```python
from build123d import *

# Parameters (mm, degrees)
BODY_START          = -127.5
SKETCH1_R           = 25
BODY_DEPTH          = 255
END_CAP_IN_START    = -127.5
SKETCH2_R           = 26
END_CAP_IN_DEPTH    = 18
END_CAP_OUT_START   = 109.5
SKETCH3_R           = 26
END_CAP_OUT_DEPTH   = 18
INLET_PORT_START    = -139.5
SKETCH4_R           = 6
INLET_PORT_DEPTH    = 12
INLET_SOCKET_START  = -139.5
SKETCH5_R           = 3.2
INLET_SOCKET_DEPTH  = 10
OUTLET_PORT_START   = 127.5
SKETCH6_R           = 6
OUTLET_PORT_DEPTH   = 12
OUTLET_SOCKET_START = 129.5
SKETCH7_R           = 3.2
OUTLET_SOCKET_DEPTH = 10


with BuildPart() as part:
    # Sketch1 → Body (new body)
    with BuildSketch(Plane(origin=(0, 0, 0), x_dir=(0, 0, -1), z_dir=(1, 0, 0)).offset(BODY_START)):
        Circle(SKETCH1_R)
    extrude(amount=BODY_DEPTH)

    # Sketch2 → End_Cap_In (add)
    with BuildSketch(Plane(origin=(0, 0, 0), x_dir=(0, 0, -1), z_dir=(1, 0, 0)).offset(END_CAP_IN_START)):
        Circle(SKETCH2_R)
    extrude(amount=END_CAP_IN_DEPTH)

    # Sketch3 → End_Cap_Out (add)
    with BuildSketch(Plane(origin=(0, 0, 0), x_dir=(0, 0, -1), z_dir=(1, 0, 0)).offset(END_CAP_OUT_START)):
        Circle(SKETCH3_R)
    extrude(amount=END_CAP_OUT_DEPTH)

    # Sketch4 → Inlet_Port (add)
    with BuildSketch(Plane(origin=(0, 0, 0), x_dir=(0, 0, -1), z_dir=(1, 0, 0)).offset(INLET_PORT_START)):
        Circle(SKETCH4_R)
    extrude(amount=INLET_PORT_DEPTH)

    # Sketch5 → Inlet_Socket (cut)
    with BuildSketch(Plane(origin=(0, 0, 0), x_dir=(0, 0, -1), z_dir=(1, 0, 0)).offset(INLET_SOCKET_START)):
        Circle(SKETCH5_R)
    extrude(amount=INLET_SOCKET_DEPTH, mode=Mode.SUBTRACT)

    # Sketch6 → Outlet_Port (add)
    with BuildSketch(Plane(origin=(0, 0, 0), x_dir=(0, 0, -1), z_dir=(1, 0, 0)).offset(OUTLET_PORT_START)):
        Circle(SKETCH6_R)
    extrude(amount=OUTLET_PORT_DEPTH)

    # Sketch7 → Outlet_Socket (cut)
    with BuildSketch(Plane(origin=(0, 0, 0), x_dir=(0, 0, -1), z_dir=(1, 0, 0)).offset(OUTLET_SOCKET_START)):
        Circle(SKETCH7_R)
    extrude(amount=OUTLET_SOCKET_DEPTH, mode=Mode.SUBTRACT)


solid = part.part
```
Source: CAD feature listing. Evaluate the final solid. Frame: model axes, mm. A direction names the side the tool comes from. Round coordinates to 2 decimals unless told otherwise and drop trailing zeros. Write each loop counter-clockwise with the first axis right and the second up, starting at its lowest first coordinate (ties: lowest second). Pieces come first, ordered by that corner, then holes. Notation, with made-up numbers: M 7.25,-29 L 53.25,-29 A32 cw 53.25,7 Z; hole C 73.25,51 d11. An arc over 180 degrees is marked long. Answer as a JSON object with one key per item and string values. Group by question number.
(1) Ray query, line 1 (Y direction, x = 133, z = 0); line 2 (X direction, y = 11, z = 23.5); line 3 (X direction, y = -17, z = -12). Return the intervals inside material, ascending. Write a range as [from, to].
(2) Section query A-A on z = 0. Output: boundary loops of the cut face in (x, y), then the cut area to 3 significant figures.
(3) First-contact query: pin 1 (12 mm diameter, centred on y = 8, z = 20, fed in from -X); pin 2 (3 mm diameter, centred on y = 0.5, z = 0, fed in from -X); pin 3 (15.5 mm diameter, centred on y = 11, z = 11, fed in from +X). Flat tips, straight axial feed; report the tip coordinate or a pass-through.
(4) Section query D-D on y = 16.5. Output: boundary loops of the cut face in (x, z), then the cut area to 3 significant figures.
(5) Section query C-C on x = 61. Output: boundary loops of the cut face in (y, z), then the cut area to 3 significant figures.
(6) Reachability of faces 1 (the flat face through (129.5, 0, 0)), 2 (the flat face through (-129.5, 0, 0)), 3 (the cylindrical face through (-118.626, -15.821, 20.633)), 4 (the flat face through (-109.5, 21, 14)) from +Z, -Z, +X, -X, +Y, -Y: full face, straight path, thin tool, end or side. Return the list, or none.
(7) Mould query, pull axis X, two halves, no side actions, for faces 5 (the flat face through (139.5, -3, -3)), 6 (the flat face through (-139.5, -3, -3)), 7 (the cylindrical face through (-1.533, 7.509, -23.846)), 8 (the flat face through (109.5, 21, 14)). Classes: +X half, -X half, draft (parallel to the pull), parting line (faces both ways), or undercut.
Computed values:
{
 "1": {"line 1": "[-6, -3.2], [3.2, 6]", "line 2": "[-127.5, -109.5], [109.5, 127.5]", "line 3": "[-127.5, 127.5]"},
 "2": {"outline": "M -139.5,-6 L -127.5,-6 L -127.5,-26 L -109.5,-26 L -109.5,-25 L 109.5,-25 L 109.5,-26 L 127.5,-26 L 127.5,-6 L 139.5,-6 L 139.5,-3.2 L 129.5,-3.2 L 129.5,3.2 L 139.5,3.2 L 139.5,6 L 127.5,6 L 127.5,26 L 109.5,26 L 109.5,25 L -109.5,25 L -109.5,26 L -127.5,26 L -127.5,6 L -139.5,6 L -139.5,3.2 L -129.5,3.2 L -129.5,-3.2 L -139.5,-3.2 Z", "area": "13,000 mm^2"},
 "3": {"pin 1": "x = -127.5", "pin 2": "x = -129.5", "pin 3": "x = 127.5"},
 "4": {"outline": "M -127.5,-20.09 L -109.5,-20.09 L -109.5,-18.78 L 109.5,-18.78 L 109.5,-20.09 L 127.5,-20.09 L 127.5,20.09 L 109.5,20.09 L 109.5,18.78 L -109.5,18.78 L -109.5,20.09 L -127.5,20.09 Z", "area": "9,670 mm^2"},
 "5": {"outline": "C 0,0 d50", "area": "1,960 mm^2"},
 "6": {"face 1": "+X", "face 2": "-X", "face 3": "+X, -X", "face 4": "none"},
 "7": {"face 5": "+X half", "face 6": "-X half", "face 7": "undercut", "face 8": "undercut"}
}
